Here's how the part is built. I have some questions about the finished solid (model axes, mm). Face numbers are marked on the shaded views. A direction names the side the tool comes from. Coordinates: 2 decimals unless noted, no trailing zeros. Order: outer loops, then holes, each group sorted by start corner. A loop starts at its lowest first (then second) coordinate and runs counter-clockwise, first axis right, second up.
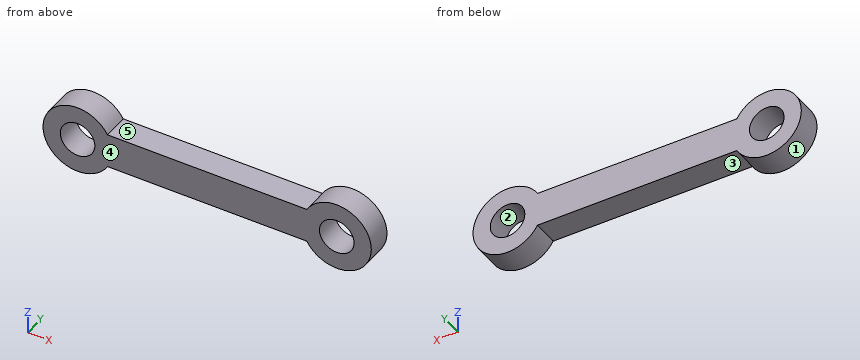
```python
from build123d import *

# Parameters (mm, degrees)
BOSS_EXTRUDE1_DEPTH = 15
F_20_0MM_1_D        = 20
SCALE_1_SCALE       = 0.3


with BuildPart() as part:
    # Sketch1 → Boss-Extrude1 (new body)
    with BuildSketch(Plane(origin=(0, 0, 0), x_dir=(1, 0, 0), z_dir=(0, 1, 0))):
        with BuildLine():
            Line((57.679491924, 10), (-57.679491924, 10))
            ThreePointArc((-57.679491924, 10), (-95, 0), (-57.679491924, -10))
            Line((-57.679491924, -10), (57.679491924, -10))
            ThreePointArc((57.679491924, -10), (95, 0), (57.679491924, 10))
        make_face()
    extrude(amount=BOSS_EXTRUDE1_DEPTH)

    # Ø20.0mm 맞춤핀 구멍1 (through all)
    with Locations(Plane(origin=(0, 15, 0), x_dir=(1, 0, 0), z_dir=(0, 1, 0))):
        with Locations((-75, 0), (75, 0)):
            Hole(F_20_0MM_1_D / 2)


with BuildPart() as part_1:
    # 축척1: scaled about (0, 7.5, 0)
    add(part.part.scale(SCALE_1_SCALE).moved(Location((0, 5.25, 0))))


solid = part_1.part
```
Q1. If we section it at C-C on y = 9: Write out the boundary of the cut face in (x, z), then the cut area to 3 significant figures.
Q2. Will these pins go through, and if not, where does the flat tip stop? pin 1 (1 mm diameter, centred on y = 6.5, z = 1.5, fed in from +X); pin 2 (1.3 mm diameter, centred on x = 5, y = 7, fed in from -Z).
Q3. If we section it at A-A on x = -22.5: Write out the boundary of the cut face in (y, z), then the cut area to 3 significant figures.
Q4. For the marked faces 4 and 5, which set-ups out of +Z, -Z, +X, -X, +Y, -Y let a thin tool reach every point of the face, with its end or its side?
Q5. If we section it at D-D on z = -4.5: Write out the boundary of the cut face in (x, y).
Q6. If we section it at B-B on z = 0: Write out the boundary of the cut face in (x, y).
Q7. We'd pull the mould along Z, two halves only. Please class the marked faces 1, 2 and 3: pulls with the +Z half, pulls with the -Z half, needs draft (parallel to the pull), parting line crosses it, or undercut.
Q8. I need wall thicknesses on L1, parallel to X at y = 7.85, z = 1.25; L2, parallel to Z at x = 22.5, y = 7.2; L3, parallel to X at y = 6.3, z = 0.75. Which ranges of each line are inside material? Lowest first, please.
Reply:
1. outline: (-17.3, -3) - (17.3, -3) arc R6 ccw (long way) to (17.3, 3) - (-17.3, 3) arc R6 ccw (long way) to start; hole circle Ø6 at (-22.5, 0); hole circle Ø6 at (22.5, 0)
1. area: 371 mm2
2. pin 1: stops at x = 28.42
2. pin 2: stops at z = -3
3. outline: (5.25, -6) - (9.75, -6) - (9.75, -3) - (5.25, -3) - close; (5.25, 3) - (9.75, 3) - (9.75, 6) - (5.25, 6) - close
3. area: 27.0 mm2
4. face 4: +Z, -Z, +X, -X, -Y
4. face 5: +Z, +Y, -Y
5. outline: (-26.47, 5.25) - (-18.53, 5.25) - (-18.53, 9.75) - (-26.47, 9.75) - close; (18.53, 5.25) - (26.47, 5.25) - (26.47, 9.75) - (18.53, 9.75) - close
6. outline: (-28.5, 5.25) - (-25.5, 5.25) - (-25.5, 9.75) - (-28.5, 9.75) - close; (-19.5, 5.25) - (19.5, 5.25) - (19.5, 9.75) - (-19.5, 9.75) - close; (25.5, 5.25) - (28.5, 5.25) - (28.5, 9.75) - (25.5, 9.75) - close
7. face 1: parting line crosses it
7. face 2: undercut
7. face 3: pulls with the -Z half
8. L1: x = -28.37 to -25.23, -19.77 to 19.77, 25.23 to 28.37
8. L2: z = -6 to -3, 3 to 6
8. L3: x = -28.45 to -25.4, -19.6 to 19.6, 25.4 to 28.45
